```python
from build123d import *

# Parameters (mm, degrees)
ESBO_O1_W                            = 150
ESBO_O1_H                            = 40
RESSALTO_EXTRUS_O1_DEPTH             = 50.8
ESBO_O2_R                            = 5.15
ESBO_O2_R_2                          = 11
CORTE_EXTRUS_O1_DEPTH                = 93.766588813
ESBO_O3_R                            = 1.75
CORTE_EXTRUS_O2_DEPTH                = 93.766588813
PADR_OCIRCULAR1_COUNT                = 4
ESBO_O5_R                            = 4
CORTE_EXTRUS_O3_DEPTH                = 100.023431571
FURO_ROSCADO_DE_M10X1_01_D           = 9
FURO_ROSCADO_DE_M10X1_01_CSINK_D     = 10.05
FURO_ROSCADO_DE_M10X1_01_CSINK_ANGLE = 90


with BuildPart() as part:
    # Esboço1 → Ressalto-extrusão1 (new body)
    with BuildSketch(Plane(origin=(0, 0, 0), x_dir=(1, 0, 0), z_dir=(0, 1, 0))):
        Rectangle(ESBO_O1_W, ESBO_O1_H)
    extrude(amount=RESSALTO_EXTRUS_O1_DEPTH)

    # Esboço2 → Corte-extrusão1 (cut, through all)
    with BuildSketch(Plane(origin=(0, 50.8, 0), x_dir=(1, 0, 0), z_dir=(0, 1, 0))):
        with Locations(Location((0, 0, 0), (0, 0, 270))):
            Circle(ESBO_O2_R)
        with Locations(Location((-57.5, 0, 0), (0, 0, 270))):
            Circle(ESBO_O2_R_2)
        with Locations(Location((57.5, 0, 0), (0, 0, 270))):
            Circle(ESBO_O2_R_2)
    extrude(amount=-CORTE_EXTRUS_O1_DEPTH, mode=Mode.SUBTRACT)

    # Esboço3 → Corte-extrusão2 (cut, through all)
    with BuildSketch(Plane(origin=(0, 50.8, 0), x_dir=(1, 0, 0), z_dir=(0, 1, 0))):
        with Locations(Location((0, 8, 0), (0, 0, 270))):
            Circle(ESBO_O3_R)
    corte_extrus_o2 = extrude(amount=-CORTE_EXTRUS_O2_DEPTH, mode=Mode.SUBTRACT)

    # PadrãoCircular1: Corte-extrusão2 ×4 about axis
    padr_ocircular1_axis = Axis((0, 0, 0), (0, 1, 0))
    for i in range(1, PADR_OCIRCULAR1_COUNT):
        add(corte_extrus_o2.rotate(padr_ocircular1_axis, i * 360 / PADR_OCIRCULAR1_COUNT), mode=Mode.SUBTRACT)

    # Esboço5 → Corte-extrusão3 (cut, through all)
    with BuildSketch(Plane(origin=(0, 0, -20), x_dir=(-1, 0, 0), z_dir=(0, 0, -1))):
        with Locations((35, 25.4)):
            Circle(ESBO_O5_R)
        with Locations((-35, 25.4)):
            Circle(ESBO_O5_R)
    extrude(amount=-CORTE_EXTRUS_O3_DEPTH, mode=Mode.SUBTRACT)

    # Furo roscado de M10x1.01 (through all)
    with Locations(Plane(origin=(0, 0, -20), x_dir=(-1, 0, 0), z_dir=(0, 0, -1))):
        with Locations((35, 25.4), (-35, 25.4)):
            CounterSinkHole(FURO_ROSCADO_DE_M10X1_01_D / 2, FURO_ROSCADO_DE_M10X1_01_CSINK_D / 2, counter_sink_angle=FURO_ROSCADO_DE_M10X1_01_CSINK_ANGLE)


solid = part.part
```
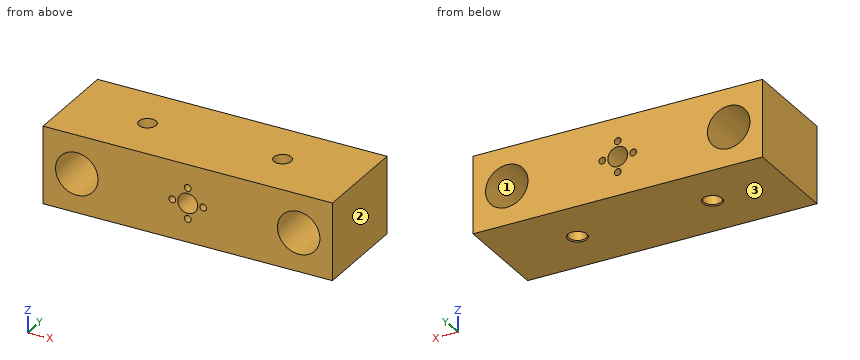
Could you check a few things on this model? Use its own coordinates, in mm. Face numbers are marked on the shaded views. Coordinates: 2 decimals unless noted, no trailing zeros. Write each loop counter-clockwise with the first axis right and the second up, starting at its lowest first coordinate (ties: lowest second). Pieces come first, ordered by that corner, then holes. Notation, with made-up numbers: (27, -13) - (78, -13) arc R20 cw to (78, 26) - close; hole circle Ø11 at (-25.5, -32). An arc over 180 degrees is marked (long way). Use a Markdown table: item, result.
Q1. Imagine slicing it at D-D (y = 9). List the corners of the cut face in (x, z) for me, and give its area (3 significant figures).
Geometry check:
| item | result |
|---|---|
| outline | (-75, -20) - (75, -20) - (75, 20) - (-75, 20) - close; hole circle Ø22 at (-57.5, 0); hole circle Ø3.5 at (-8, 0); hole circle Ø10.3 at (0, 0); hole circle Ø3.5 at (0, -8); hole circle Ø3.5 at (0, 8); hole circle Ø3.5 at (8, 0); hole circle Ø22 at (57.5, 0) |
| area | 5,120 mm2 |
Q2. Imagine slicing it at B-B (x = -57.5). List the corners of the cut face in (y, z) for me, and give its area (3 significant figures).
Geometry check:
| item | result |
|---|---|
| outline | (0, -20) - (50.8, -20) - (50.8, -11) - (0, -11) - close; (0, 11) - (50.8, 11) - (50.8, 20) - (0, 20) - close |
| area | 914 mm2 |
Q3. Thinking about a two-plate mould opening in Z: for the marked faces 1, 2 and 3, which applies, +Z half, -Z half, draft (parallel to the pull), parting line (faces both ways), or undercut?
Geometry check:
| item | result |
|---|---|
| face 1 | undercut |
| face 2 | draft |
| face 3 | -Z half |
Q4. Please list where these lines run through material, in increasing order: L1, parallel to Z at x = -57, y = 30; L2, parallel to X at y = 11, z = 6.5; L3, parallel to X at y = 25.4, z = 2.
Geometry check:
| item | result |
|---|---|
| L1 | z = -20 to -10.99, 10.99 to 20 |
| L2 | x = -75 to -66.37, -48.63 to -0.9, 0.9 to 48.63, 66.37 to 75 |
| L3 | x = -75 to -68.32, -46.68 to -39.5, -30.5 to -4.75, 4.75 to 30.5, 39.5 to 46.68, 68.32 to 75 |
Q5. Imagine slicing it at C-C (z = 8). List the corners of the cut face in (x, y) for me, and give its area (3 significant figures).
Geometry check:
| item | result |
|---|---|
| outline | (-75, 0) - (-65.05, 0) - (-65.05, 50.8) - (-75, 50.8) - close; (-49.95, 0) - (-1.75, 0) - (-1.75, 50.8) - (-49.95, 50.8) - close; (1.75, 0) - (49.95, 0) - (49.95, 50.8) - (1.75, 50.8) - close; (65.05, 0) - (75, 0) - (75, 50.8) - (65.05, 50.8) - close; hole circle Ø9 at (-35, 25.4); hole circle Ø9 at (35, 25.4) |
| area | 5,780 mm2 |
Q6. Imagine slicing it at A-A (y = 25.4). Count the separate pieces of the cut face and the enclosed holes in it, and give its area (3 significant figures).
Geometry check:
| item | result |
|---|---|
| separate pieces | 3 |
| enclosed holes | 7 |
| area | 4,400 mm2 |
Q7. I'm going to push a flat-ended pin straight in: pin 1 Ø17.5 at (x, z) = (57.5, 0) entering from -Y. Where does the tip first touch, or does it pass through?
Geometry check:
| item | result |
|---|---|
| pin 1 | passes through |
